The listing builds one solid part. Answer for the finished solid, in the listing's coordinates (mm). A direction names the side the tool comes from. Round coordinates to 2 decimals unless told otherwise and drop trailing zeros. Write each loop counter-clockwise with the first axis right and the second up, starting at its lowest first coordinate (ties: lowest second). Pieces come first, ordered by that corner, then holes.
Item 1: Find section B-B on y = 7.5. Give the vertices of the cut face in (x, z).
Item 2: Find the intervals of material crossed by probe 1 along Z at (x, y) = (-5, 7.75); probe 2 along X at (y, z) = (0.5, 1.75), in increasing order.
Item 3: A tool of negligible diameter and unlimited length cuts with its end or side. For faces 5 (the face through (-1.2, 0, 7.3)), 6 (the face through (14.25, 6, 0)), from which of +Z, -Z, +X, -X, +Y, -Y can it reach the whole face along a straight path? Write none if from no direction.
Item 4: Find section A-A on x = -11. Give the vertices of the cut face in (y, z), then the cut area to 3 significant figures.
Item 5: Find section C-C on z = 5. Give the vertices of the cut face in (x, y).
Item 6: For a pull along X with two mould halves and no side action, classify faces 1 (the face through (-15.75, 6, 0)), 2 (the face through (0, 6, 7)), 3 (the face through (0, 6, -7)), 4 (the face through (0, 6, -8.25)) as +X half, -X half, draft (parallel to the pull), parting line (faces both ways), or undercut.
Item 7: This flat-tipped pin is pushed along its axis until it touches: pin 1 (1.5 mm diameter, centred on x = 3.5, z = -6, fed in from +Y). Where does it stop, or does it pass through?
```python
from build123d import *

# Parameters (mm, degrees)
SKETCH1_W           = 31.5
SKETCH1_H           = 16.5
BOSS_EXTRUDE1_DEPTH = 13
SKETCH2_W           = 21.5
SKETCH2_H           = 2
CUT_EXTRUDE1_DEPTH  = 14


with BuildPart() as part:
    # Sketch1 → Boss-Extrude1 (new body)
    with BuildSketch(Plane(origin=(0, 0, 0), x_dir=(1, 0, 0), z_dir=(0, 1, 0))):
        Rectangle(SKETCH1_W, SKETCH1_H)
        Polygon((10.75, 5), (-10.75, 5), (-10.75, 7), (-14.25, 7), (-14.25, -7), (-10.75, -7), (-10.75, -5), (10.75, -5), (10.75, -7), (14.25, -7), (14.25, 7), (10.75, 7), align=None, mode=Mode.SUBTRACT)
    extrude(amount=BOSS_EXTRUDE1_DEPTH)

    # Sketch2 → Cut-Extrude1 (cut, through all)
    with BuildSketch(Plane.XZ):
        with Locations((0, 6)):
            Rectangle(SKETCH2_W, SKETCH2_H)
        with Locations((0, -6)):
            Rectangle(SKETCH2_W, SKETCH2_H)
    extrude(amount=-CUT_EXTRUDE1_DEPTH, mode=Mode.SUBTRACT)


solid = part.part
```
Check values:
1. outline: (-15.75, -8.25) - (15.75, -8.25) - (15.75, 8.25) - (-15.75, 8.25) - close; hole (-14.25, -7) - (14.25, -7) - (14.25, 7) - (-14.25, 7) - close
2. probe 1: z = -8.25 to -7, 7 to 8.25
2. probe 2: x = -15.75 to -14.25, 14.25 to 15.75
3. face 5: +Z, -Z, +X, -X, -Y
3. face 6: +Y, -Y
4. outline: (0, -8.25) - (13, -8.25) - (13, -7) - (0, -7) - close; (0, 7) - (13, 7) - (13, 8.25) - (0, 8.25) - close
4. area: 32.5 mm2
5. outline: (-15.75, 0) - (-14.25, 0) - (-14.25, 13) - (-15.75, 13) - close; (14.25, 0) - (15.75, 0) - (15.75, 13) - (14.25, 13) - close
6. face 1: -X half
6. face 2: undercut
6. face 3: undercut
6. face 4: draft
7. pin 1: passes through
